from build123d import *

# Parameters (mm, degrees)
F1_DEPTH = 25.4


with BuildPart() as f1:
    # F0 (on Front) → F1 (new body)
    with BuildSketch(Plane.XZ):
        with BuildLine():
            ThreePointArc((-89.08151, 23.215859), (-73.927081, -13.413316), (-42.474968, 10.713801))
            ThreePointArc((-42.474968, 10.713801), (-50.259571, 28.833407), (-68.761512, 35.659704))
            ThreePointArc((-68.761512, 35.659704), (-80.500818, 32.016689), (-89.08151, 23.215859))
        make_face()
        with BuildLine():
            ThreePointArc((-89.08151, 23.215859), (-80.500818, 32.016689), (-68.761512, 35.659704))
            Line((-68.761512, 35.659704), (-68.761512, 41.479227))
            ThreePointArc((-68.761512, 41.479227), (-9.89729, 100.779416), (49.835637, 42.354366))
            Line((49.835637, 42.354366), (49.835637, 36.492049))
            ThreePointArc((49.835637, 36.492049), (61.077606, 34.522835), (70.371209, 27.897986))
            Line((70.371209, 27.897986), (70.153422, 42.654235))
            ThreePointArc((70.153422, 42.654235), (-10.047229, 121.098861), (-89.08151, 41.479227))
            Line((-89.08151, 41.479227), (-89.08151, 23.215859))
        make_face()
        with BuildLine():
            ThreePointArc((70.371209, 27.897986), (61.077606, 34.522835), (49.835637, 36.492049))
            ThreePointArc((49.835637, 36.492049), (33.320821, -7.982932), (76.923518, 10.713801))
            ThreePointArc((76.923518, 10.713801), (75.229873, 19.909302), (70.371209, 27.897986))
        make_face()
    extrude(amount=F1_DEPTH)


solid = f1.part
Can you work these out from the model? Positions are in its coordinate system, mm. A direction names the side the tool comes from. Round coordinates to 2 decimals unless told otherwise and drop trailing zeros. Loops run counter-clockwise (first coordinate to the right, second up) from the corner with the lowest first, then second, coordinate; pieces in that order, holes last. Notation, with made-up numbers: (75, -26.5) - (113, -26.5) arc R38 ccw to (113, 12.5) - close; hole circle Ø3 at (49.5, 79). An arc over 180 degrees is marked (long way). Use CSV: the item, a comma, the result in double quotes. Start each with the question number.
1) Please list where these lines run through material, in increasing order: probe 1 along X at (y, z) = (-6, 43); probe 2 along X at (y, z) = (-3.25, 42); probe 3 along Z at (x, y) = (32, -1.25). Write a range as [from, to].
2) We'd pull the mould along X, two halves only. Please class faces 1 (the flat face through (-47, -25.4, 24)), 2 (the flat face through (-68.762, -13, 39)), 3 (the flat face through (-89.082, -13, 32)): released by +X, released by -X, zero draft, split by the parting line, or undercut.
3) If we section it at C-C on x = -58.5: Write out the boundary of the cut face in (y, z), plus the area to 3 significant figures.
4) For faces 4 (the cylindrical face through (-11.195, -12.522, 100.756)), 5 (the cylindrical face through (-8.305, -12.522, 121.093)), which set-ups out of +Z, -Z, +X, -X, +Y, -Y let a thin tool reach every point of the face, with its end or its side?
5) For pin 1 Ø1 at (x, y) = (-73.5, -5.5) entering from -Z; pin 2 Ø4.5 at (y, z) = (-9.5, 37.5) entering from +X; pin 3 Ø12 at (y, z) = (-11.5, 63.5) entering from +X, each with a flat end and sliding along its axis, tell me the tip position at first contact or that it passes through.
6) If we section it at A-A on z = 45: Write out the boundary of the cut face in (x, y).
7) If we section it at D-D on x = -21: Write out the boundary of the cut face in (y, z), plus the area to 3 significant figures.
Geometry results:
1,probe 1,"x = [-89.07, -68.74], [49.82, 70.15]"
1,probe 2,"x = [-89.08, -68.76], [49.84, 70.16]"
1,probe 3,"z = [-6.63, 28.06], [83.88, 109.46]"
2,face 1,"zero draft"
2,face 2,"undercut"
2,face 3,"released by -X"
3,outline,"(-25.4, -12.61) - (0, -12.61) - (0, 34.03) - (-25.4, 34.03) - close; (-25.4, 74.82) - (0, 74.82) - (0, 104.21) - (-25.4, 104.21) - close"
3,area,"1,930 mm2"
4,face 4,"+Y, -Y"
4,face 5,"+Z, +Y, -Y"
5,pin 1,"stops at z = -13.64"
5,pin 2,"stops at x = 70.26"
5,pin 3,"stops at x = 68.53"
6,outline,"(-89, -25.4) - (-68.66, -25.4) - (-68.66, 0) - (-89, 0) - close; (49.74, -25.4) - (70.08, -25.4) - (70.08, 0) - (49.74, 0) - close"
7,outline,"(-25.4, 99.65) - (0, 99.65) - (0, 120.26) - (-25.4, 120.26) - close"
7,area,"524 mm2"
